from build123d import *

# Parameters (mm, degrees)
CUT_EXTRUDE1_DEPTH = 5
SKETCH3_W          = 6
SKETCH3_H          = 5
CUT_EXTRUDE2_DEPTH = 12


with BuildPart() as part:
    # Sketch1 → Revolve1 (revolve)
    with BuildSketch(Plane(origin=(0, 0, 0), x_dir=(0, 0, -1), z_dir=(1, 0, 0))):
        Polygon((0, 0), (0, 6.5), (20, 6.5), (25, 5.5), (25, 0), align=None)
    revolve(axis=Axis((0, 0, -25), (0, 0, 1)))

    # Sketch2 → Cut-Extrude1 (cut)
    with BuildSketch(Plane(origin=(0, 0, -25), x_dir=(-1, 0, 0), z_dir=(0, 0, -1))):
        with BuildLine():
            Line((-3, 5.766281297), (-3, -5.766281297))
            ThreePointArc((-3, -5.766281297), (-6.5, 0), (-3, 5.766281297))
        make_face()
        with BuildLine():
            Line((3, 5.766281297), (3, -5.766281297))
            ThreePointArc((3, -5.766281297), (6.5, 0), (3, 5.766281297))
        make_face()
    extrude(amount=-CUT_EXTRUDE1_DEPTH, mode=Mode.SUBTRACT)

    # Sketch3 → Cut-Extrude2 (cut)
    with BuildSketch(Plane(origin=(0, 0, -20), x_dir=(-1, 0, 0), z_dir=(0, 0, -1))):
        with Locations((6.5, 0)):
            Rectangle(SKETCH3_W, SKETCH3_H)
    extrude(amount=-CUT_EXTRUDE2_DEPTH, mode=Mode.SUBTRACT)


solid = part.part
Work out the finished part from the listing and answer in its coordinate system (mm). A direction names the side the tool comes from. Give positions to 0.01 mm unless a question says otherwise; leave off trailing zeros. Write each loop counter-clockwise with the first axis right and the second up, starting at its lowest first coordinate (ties: lowest second). Pieces come first, ordered by that corner, then holes.
Q1. The part is cut by section B-B on x = -5.5. Give the vertices of the cut face in (y, z).
Answer:
outline: (-3.46, -20) - (-2.5, -20) - (-2.5, -8) - (2.5, -8) - (2.5, -20) - (3.46, -20) - (3.46, 0) - (-3.46, 0) - close
Q2. For a pull along Y with two mould halves and no side action, classify faces 1 (the face through (0, 6, -22.5)), 2 (the face through (0, 0, -25)), 3 (the face through (-5, 0, -8)) as released by +Y, released by -Y, zero draft, split by the parting line, or undercut.
Answer:
face 1: released by +Y
face 2: zero draft
face 3: undercut
Q3. The part is cut by section C-C on z = -6.5. Give the vertices of the cut face in (x, y), and give its area (3 significant figures).
Answer:
outline: circle Ø13 at (0, 0)
area: 133 mm2
Q4. Straight lines are drawn through the part: L1, parallel to Z at x = 4, y = 2.75; L2, parallel to X at y = -3, z = -5; L3, parallel to Z at x = -4.25, y = -1.5. For each, find the intervals that lie inside material, in ascending order.
Answer:
L1: z = -20 to 0
L2: x = -5.77 to 5.77
L3: z = -8 to 0
Q5. The part is cut by section A-A on y = 0. Give the vertices of the cut face in (x, z), and give its area (3 significant figures).
Answer:
outline: (-6.5, -8) - (-3.5, -8) - (-3.5, -20) - (-3, -20) - (-3, -25) - (3, -25) - (3, -20) - (6.5, -20) - (6.5, 0) - (-6.5, 0) - close
area: 254 mm2
Q6. Given pin 1 (0.9 mm diameter, centred on x = -5, y = -0.5, fed in from -Z); pin 2 (0.8 mm diameter, centred on x = -5, z = -14.5, fed in from -Y); pin 3 (5.5 mm diameter, centred on y = -1.5, z = -22, fed in from +X); pin 4 (4 mm diameter, centred on y = -2, z = -23.5, fed in from -X), each flat-ended and moving along its own axis, determine where each tip first touches the part or whether it passes through.
Answer:
pin 1: stops at z = -8
pin 2: stops at y = -4.59
pin 3: stops at x = 6.5
pin 4: stops at x = -3
Q7. A tool of negligible diameter and unlimited length cuts with its end or side. For faces 4 (the face through (-5, 2.5, -14)), 5 (the face through (-3, 0, -23)), 6 (the face through (4, 0, -20)), from which of +Z, -Z, +X, -X, +Y, -Y can it reach the whole face along a straight path? Write none if from no direction.
Answer:
face 4: -Z, -X
face 5: -Z, -X, +Y, -Y
face 6: -Z, +X, +Y, -Y
Q8. The part is cut by section D-D on x = -4. Give the vertices of the cut face in (y, z), and give its area (3 significant figures).
Answer:
outline: (-5.12, -20) - (-2.5, -20) - (-2.5, -8) - (2.5, -8) - (2.5, -20) - (5.12, -20) - (5.12, 0) - (-5.12, 0) - close
area: 145 mm2
